from build123d import *

# Parameters (mm, degrees)
SKETCH1_W           = 110
SKETCH1_H           = 45.5
BOSS_EXTRUDE1_DEPTH = 2
CUT_EXTRUDE1_REACH  = 61.553
SKETCH2_R           = 1.5
SKETCH2_W           = 7.5
SKETCH2_H           = 20


with BuildPart() as part:
    # Sketch1 → Boss-Extrude1 (new body)
    with BuildSketch(Plane(origin=(0, 0, 0), x_dir=(1, 0, 0), z_dir=(0, 1, 0))):
        Rectangle(SKETCH1_W, SKETCH1_H)
    extrude(amount=BOSS_EXTRUDE1_DEPTH)

    # Sketch2 → Cut-Extrude1 (cut, up to next)
    with BuildSketch(Plane(origin=(0, 2, 0), x_dir=(1, 0, 0), z_dir=(0, 1, 0)), mode=Mode.PRIVATE) as cut_extrude1_sk1:
        with Locations(Location((-46, -13.75, 0), (0, 0, 270))):
            Circle(SKETCH2_R)
    cut_extrude1_tool1 = extrude(cut_extrude1_sk1.sketch, amount=-CUT_EXTRUDE1_REACH, mode=Mode.PRIVATE) & part.part
    # Sketch2 → Cut-Extrude1 (cut, up to next)
    with BuildSketch(Plane(origin=(0, 2, 0), x_dir=(1, 0, 0), z_dir=(0, 1, 0)), mode=Mode.PRIVATE) as cut_extrude1_sk2:
        with Locations(Location((-46, 13.75, 0), (0, 0, 270))):
            Circle(SKETCH2_R)
    cut_extrude1_tool2 = extrude(cut_extrude1_sk2.sketch, amount=-CUT_EXTRUDE1_REACH, mode=Mode.PRIVATE) & part.part
    # Sketch2 → Cut-Extrude1 (cut, up to next)
    with BuildSketch(Plane(origin=(0, 2, 0), x_dir=(1, 0, 0), z_dir=(0, 1, 0)), mode=Mode.PRIVATE) as cut_extrude1_sk3:
        with Locations(Location((46, 13.75, 0), (0, 0, 270))):
            Circle(SKETCH2_R)
    cut_extrude1_tool3 = extrude(cut_extrude1_sk3.sketch, amount=-CUT_EXTRUDE1_REACH, mode=Mode.PRIVATE) & part.part
    # Sketch2 → Cut-Extrude1 (cut, up to next)
    with BuildSketch(Plane(origin=(0, 2, 0), x_dir=(1, 0, 0), z_dir=(0, 1, 0)), mode=Mode.PRIVATE) as cut_extrude1_sk4:
        with Locations(Location((46, -13.75, 0), (0, 0, 270))):
            Circle(SKETCH2_R)
    cut_extrude1_tool4 = extrude(cut_extrude1_sk4.sketch, amount=-CUT_EXTRUDE1_REACH, mode=Mode.PRIVATE) & part.part
    # Sketch2 → Cut-Extrude1 (cut, up to next)
    with BuildSketch(Plane(origin=(0, 2, 0), x_dir=(1, 0, 0), z_dir=(0, 1, 0)), mode=Mode.PRIVATE) as cut_extrude1_sk5:
        with Locations((36.25, 0)):
            Rectangle(SKETCH2_W, SKETCH2_H)
    cut_extrude1_tool5 = extrude(cut_extrude1_sk5.sketch, amount=-CUT_EXTRUDE1_REACH, mode=Mode.PRIVATE) & part.part
    add(cut_extrude1_tool1.solids().sort_by_distance((-46, 2, 13.75))[0], mode=Mode.SUBTRACT)
    add(cut_extrude1_tool2.solids().sort_by_distance((-46, 2, -13.75))[0], mode=Mode.SUBTRACT)
    add(cut_extrude1_tool3.solids().sort_by_distance((46, 2, -13.75))[0], mode=Mode.SUBTRACT)
    add(cut_extrude1_tool4.solids().sort_by_distance((46, 2, 13.75))[0], mode=Mode.SUBTRACT)
    add(cut_extrude1_tool5.solids().sort_by_distance((36.25, 2, 0))[0], mode=Mode.SUBTRACT)


solid = part.part
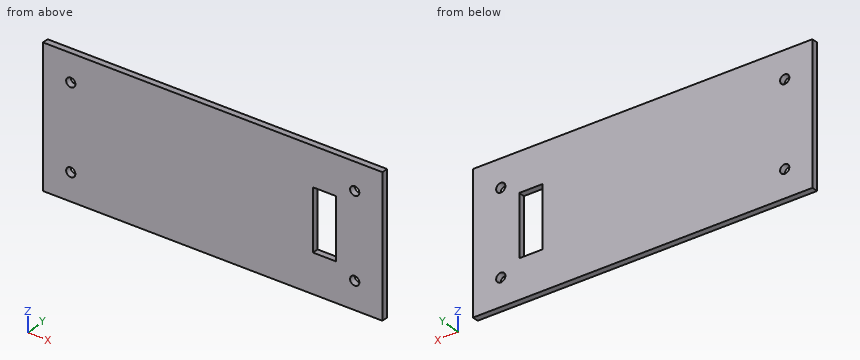
Geometry check sheet. Reference: the model listing, model coordinates, mm. Give positions to 0.01 mm unless a question says otherwise; leave off trailing zeros. Loops run counter-clockwise (first coordinate to the right, second up) from the corner with the lowest first, then second, coordinate; pieces in that order, holes last. Notation, with made-up numbers: (65, 87) -> (78, 87) arc R33 ccw to (78, 118) -> close; hole circle Ø4 at (-40, 29). An arc over 180 degrees is marked (long way). Answer in a Markdown table with one row per item. Add a question column.
1) Material ranges on probe 1 along X at (y, z) = (0.8, -13.75); probe 2 along X at (y, z) = (1.1, -4); probe 3 along X at (y, z) = (0.4, -14.5), recorded low to high. Write a range as from..to.
2) Cross-section at B-B on z = 3. Record the boundary of the cut face in (x, y), and give its area (3 significant figures).
3) Cross-section at A-A on x = 38.5. Record the boundary of the cut face in (y, z).
4) Cross-section at C-C on y = 0.55. Record the boundary of the cut face in (x, z), and give its area (3 significant figures).
5) Cross-section at D-D on x = -46. Record the boundary of the cut face in (y, z), and give its area (3 significant figures).
6) Gauge pin test, flat end, axial feed: P1, Ø3.5, axis at x = -46, z = 13.75, coming from the -Y side. Record the tip position at first contact, or that the pin passes through.
Outcome:
| question | item | result |
|---|---|---|
| 1 | probe 1 | x = -55..-47.5, -44.5..44.5, 47.5..55 |
| 1 | probe 2 | x = -55..32.5, 40..55 |
| 1 | probe 3 | x = -55..-47.3, -44.7..44.7, 47.3..55 |
| 2 | outline | (-55, 0) -> (32.5, 0) -> (32.5, 2) -> (-55, 2) -> close; (40, 0) -> (55, 0) -> (55, 2) -> (40, 2) -> close |
| 2 | area | 205 mm^2 |
| 3 | outline | (0, -22.75) -> (2, -22.75) -> (2, -10) -> (0, -10) -> close; (0, 10) -> (2, 10) -> (2, 22.75) -> (0, 22.75) -> close |
| 4 | outline | (-55, -22.75) -> (55, -22.75) -> (55, 22.75) -> (-55, 22.75) -> close; hole circle Ø3 at (-46, -13.75); hole circle Ø3 at (-46, 13.75); hole (32.5, -10) -> (40, -10) -> (40, 10) -> (32.5, 10) -> close; hole circle Ø3 at (46, -13.75); hole circle Ø3 at (46, 13.75) |
| 4 | area | 4,830 mm^2 |
| 5 | outline | (0, -22.75) -> (2, -22.75) -> (2, -15.25) -> (0, -15.25) -> close; (0, -12.25) -> (2, -12.25) -> (2, 12.25) -> (0, 12.25) -> close; (0, 15.25) -> (2, 15.25) -> (2, 22.75) -> (0, 22.75) -> close |
| 5 | area | 79.0 mm^2 |
| 6 | P1 | stops at y = 0 |
